```python
from build123d import *

# Parameters (mm, degrees)
F2_DEPTH  = 18.5
F3_R      = 1.55
F4_DEPTH  = 3.075
F5_W      = 6
F5_H      = 0.5
F6_DEPTH  = 0.2
F5_W_2    = 4
F5_H_2    = 2.25
F7_DEPTH  = 0.6
F8_W      = 4
F8_H      = 0.5
F9_DEPTH  = 0.9
F8_H_2    = 0.47
F10_DEPTH = 0.2
F11_W     = 4
F11_H     = 0.5
F12_DEPTH = 0.9
F11_H_2   = 0.47
F13_DEPTH = 0.2
F14_W     = 4
F14_H     = 0.5
F15_DEPTH = 0.7
F16_W     = 8
F16_H     = 7
F17_DEPTH = 1
F17_TAPER = 45
F18_W     = 8
F18_H     = 7
F19_DEPTH = 1
F19_TAPER = 45
F22_DEPTH = 0.2
F23_ANGLE = 90


with BuildPart() as f2:
    # F1 (on Front) → F2 (new body)
    with BuildSketch(Plane.XZ):
        with BuildLine():
            Line((-33.5725, -6), (33.5725, -6))
            ThreePointArc((33.5725, -6), (34.6331601718, -5.5606601718), (35.0725, -4.5))
            Line((35.0725, -4.5), (35.0725, 4.5))
            ThreePointArc((35.0725, 4.5), (34.6331601718, 5.5606601718), (33.5725, 6))
            Line((33.5725, 6), (-33.5725, 6))
            ThreePointArc((-33.5725, 6), (-34.6331601718, 5.5606601718), (-35.0725, 4.5))
            Line((-35.0725, 4.5), (-35.0725, -4.5))
            ThreePointArc((-35.0725, -4.5), (-34.6331601718, -5.5606601718), (-33.5725, -6))
        make_face()
        with BuildLine():
            ThreePointArc((-14.9225, -0.925), (-15.5082864376, -2.3392135624), (-16.9225, -2.925))
            Line((-16.9225, -2.925), (-30.0725, -2.925))
            ThreePointArc((-30.0725, -2.925), (-31.4867135624, -2.3392135624), (-32.0725, -0.925))
            Line((-32.0725, -0.925), (-32.0725, 0.925))
            ThreePointArc((-32.0725, 0.925), (-31.4867135624, 2.3392135624), (-30.0725, 2.925))
            Line((-30.0725, 2.925), (-16.9225, 2.925))
            ThreePointArc((-16.9225, 2.925), (-15.5082864376, 2.3392135624), (-14.9225, 0.925))
            Line((-14.9225, 0.925), (-14.9225, -0.925))
        make_face(mode=Mode.SUBTRACT)
        with BuildLine():
            Line((-9.6675, 4.265), (-1.0875, 4.265))
            ThreePointArc((-1.0875, 4.265), (-0.0268398282, 3.8256601718), (0.4125, 2.765))
            Line((0.4125, 2.765), (0.4125, -2.765))
            ThreePointArc((0.4125, -2.765), (-0.0268398282, -3.8256601718), (-1.0875, -4.265))
            Line((-1.0875, -4.265), (-9.6675, -4.265))
            ThreePointArc((-9.6675, -4.265), (-10.7281601718, -3.8256601718), (-11.1675, -2.765))
            Line((-11.1675, -2.765), (-11.1675, 2.765))
            ThreePointArc((-11.1675, 2.765), (-10.7281601718, 3.8256601718), (-9.6675, 4.265))
        make_face(mode=Mode.SUBTRACT)
        with BuildLine():
            Line((4.3325, 4.265), (12.9125, 4.265))
            ThreePointArc((12.9125, 4.265), (13.9731601718, 3.8256601718), (14.4125, 2.765))
            Line((14.4125, 2.765), (14.4125, -2.765))
            ThreePointArc((14.4125, -2.765), (13.9731601718, -3.8256601718), (12.9125, -4.265))
            Line((12.9125, -4.265), (4.3325, -4.265))
            ThreePointArc((4.3325, -4.265), (3.2718398282, -3.8256601718), (2.8325, -2.765))
            Line((2.8325, -2.765), (2.8325, 2.765))
            ThreePointArc((2.8325, 2.765), (3.2718398282, 3.8256601718), (4.3325, 4.265))
        make_face(mode=Mode.SUBTRACT)
        with BuildLine():
            ThreePointArc((32.0725, -3.8), (32.0139213562, -3.9414213562), (31.8725, -4))
            Line((31.8725, -4), (17.0725, -4))
            ThreePointArc((17.0725, -4), (16.9310786438, -3.9414213562), (16.8725, -3.8))
            Line((16.8725, -3.8), (16.8725, 3.8))
            ThreePointArc((16.8725, 3.8), (16.9310786438, 3.9414213562), (17.0725, 4))
            Line((17.0725, 4), (31.8725, 4))
            ThreePointArc((31.8725, 4), (32.0139213562, 3.9414213562), (32.0725, 3.8))
            Line((32.0725, 3.8), (32.0725, -3.8))
        make_face(mode=Mode.SUBTRACT)
    extrude(amount=-F2_DEPTH)

    # F3 (on face) → F4 (cut, through all)
    with BuildSketch(Plane.XY.offset(6)):
        with Locations((-23.4975, 13.2)):
            Circle(F3_R)
    extrude(amount=-F4_DEPTH, mode=Mode.SUBTRACT)

    # F5 (on face) → F6 (join)
    with BuildSketch(Plane.XY.offset(-2.925)):
        with Locations((-23.4975, 18.25)):
            Rectangle(F5_W, F5_H)
    extrude(amount=F6_DEPTH)

    # F5 (on face) → F7 (join)
    with BuildSketch(Plane.XY.offset(-2.925)):
        with Locations((-23.4975, 6.575)):
            Rectangle(F5_W_2, F5_H_2)
    extrude(amount=F7_DEPTH)

    # F8 (on face) → F9 (join)
    with BuildSketch(Plane.XY.offset(-4.265)):
        with Locations((-5.3775, 18.25)):
            Rectangle(F8_W, F8_H)
    extrude(amount=F9_DEPTH)

    # F8 (on face) → F10 (join)
    with BuildSketch(Plane.XY.offset(-4.265)):
        with Locations((-5.3775, 0.235)):
            Rectangle(F8_W, F8_H_2)
    extrude(amount=F10_DEPTH)

    # F11 (on face) → F12 (join)
    with BuildSketch(Plane.XY.offset(-4.265)):
        with Locations((8.6225, 18.25)):
            Rectangle(F11_W, F11_H)
    extrude(amount=F12_DEPTH)

    # F11 (on face) → F13 (join)
    with BuildSketch(Plane.XY.offset(-4.265)):
        with Locations((8.6225, 0.235)):
            Rectangle(F11_W, F11_H_2)
    extrude(amount=F13_DEPTH)

    # F14 (on face) → F15 (join)
    with BuildSketch(Plane.XY.offset(-4)):
        with Locations((24.4725, 18.25)):
            Rectangle(F14_W, F14_H)
    extrude(amount=F15_DEPTH)

    # F16 (on face) → F17 (cut)
    with BuildSketch(Plane.YZ.offset(35.0725)):
        with Locations((9.25, 0)):
            Rectangle(F16_W, F16_H)
    extrude(amount=-F17_DEPTH, taper=F17_TAPER, mode=Mode.SUBTRACT)

    # F18 (on face) → F19 (cut)
    with BuildSketch(Plane(origin=(-35.0725, 0, 0), x_dir=(0, -1, 0), z_dir=(-1, 0, 0))):
        with Locations((-9.25, 0)):
            Rectangle(F18_W, F18_H)
    extrude(amount=-F19_DEPTH, taper=F19_TAPER, mode=Mode.SUBTRACT)

    # F21 (on face) → F22 (join)
    with BuildSketch(Plane(origin=(0, 18.5, 0), x_dir=(-1, 0, 0), z_dir=(0, 1, 0))):
        with BuildLine():
            Line((-33.5725, 6), (-31.6655044446, 6))
            ThreePointArc((-31.6655044446, 6), (-36.7544805153, 7.6819805153), (-35.0725, 2.5930044446))
            Line((-35.0725, 2.5930044446), (-35.0725, 4.5))
            ThreePointArc((-35.0725, 4.5), (-34.6331601718, 5.5606601718), (-33.5725, 6))
        make_face()
        with BuildLine():
            Line((-35.0725, -4.5), (-35.0725, -2.5930044446))
            ThreePointArc((-35.0725, -2.5930044446), (-36.7544805153, -7.6819805153), (-31.6655044446, -6))
            Line((-31.6655044446, -6), (-33.5725, -6))
            ThreePointArc((-33.5725, -6), (-34.6331601718, -5.5606601718), (-35.0725, -4.5))
        make_face()
        with BuildLine():
            ThreePointArc((37.6331601718, 5.5606601718), (34.8534245792, 8.5525631767), (31.6655044446, 6))
            Line((31.6655044446, 6), (33.5725, 6))
            ThreePointArc((33.5725, 6), (34.6331601718, 5.5606601718), (35.0725, 4.5))
            Line((35.0725, 4.5), (35.0725, 2.5930044446))
            ThreePointArc((35.0725, 2.5930044446), (36.9045055313, 3.6008157245), (37.6331601718, 5.5606601718))
        make_face()
        with BuildLine():
            ThreePointArc((37.6331601718, -5.5606601718), (36.9045055313, -3.6008157245), (35.0725, -2.5930044446))
            Line((35.0725, -2.5930044446), (35.0725, -4.5))
            ThreePointArc((35.0725, -4.5), (34.6331601718, -5.5606601718), (33.5725, -6))
            Line((33.5725, -6), (31.6655044446, -6))
            ThreePointArc((31.6655044446, -6), (34.8534245792, -8.5525631767), (37.6331601718, -5.5606601718))
        make_face()
    extrude(amount=-F22_DEPTH)


with BuildPart() as f2_1:
    # F23: moved
    add(f2.part.rotate(Axis((0, 18.5, 6), (-1, 0, 0)), F23_ANGLE))


solid = f2_1.part
```
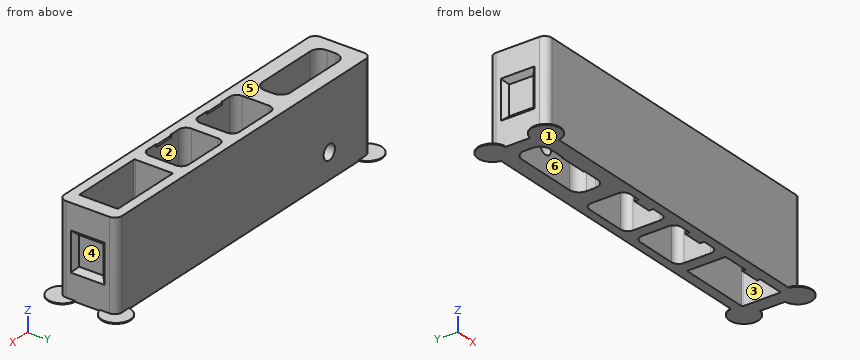
Could you check a few things on this model? Use its own coordinates, in mm. Face numbers are marked on the shaded views. A direction names the side the tool comes from. Round coordinates to 2 decimals unless told otherwise and drop trailing zeros. Loops run counter-clockwise (first coordinate to the right, second up) from the corner with the lowest first, then second, coordinate; pieces in that order, holes last. Notation, with made-up numbers: (86, 33.5) - (100, 33.5) arc R20 cw to (100, 72.5) - close; hole circle Ø3 at (42.25, 33.5). An arc over 180 degrees is marked (long way). Answer in a Markdown table with one row per item. Add a question column.
(1) For the marked faces 1, 2 and 3, which set-ups out of +Z, -Z, +X, -X, +Y, -Y let a thin tool reach every point of the face, with its end or its side?
(2) I'm going to push flat-ended pins straight in: pin 1 (9.5 mm diameter, centred on x = 6.5, z = 11, fed in from +Y); pin 2 (7.5 mm diameter, centred on x = 27, z = 19.5, fed in from -Y); pin 3 (6 mm diameter, centred on y = 6, z = 19.5, fed in from -X). Where does each tip first touch, or does it pass through?
(3) If we section it at B-B (x = 5): Please give me the cut outline in (y, z) (3 decimals).
(4) If we section it at C-C (z = 22.75): State how many separate pieces and enclosed holes the cut face has, plus the area to 3 significant figures.
(5) I need wall thicknesses on line 1 along X through (y, z) = (13.25, 17.25); line 2 along X through (y, z) = (10.25, 14.5); line 3 along Y through (x, z) = (-1.5, 21.25) (3 decimals). Which ranges of each line are inside material? Lowest first, please.
(6) If we section it at A-A (x = 30.5): Please give me the cut outline in (y, z), plus the area to 3 significant figures.
(7) If we mould it in two halves opening along X, with no side actions, what happens to the marked faces 4, 5 and 6? For each: pulls with the +X half, pulls with the -X half, needs draft (parallel to the pull), parting line crosses it, or undercut.
Model answer:
| question | item | result |
|---|---|---|
| 1 | face 1 | -Z, +X, -X, +Y, -Y |
| 1 | face 2 | none |
| 1 | face 3 | +Z, -Z |
| 2 | pin 1 | stops at y = 18.5 |
| 2 | pin 2 | stops at y = 6.5 |
| 2 | pin 3 | stops at x = -35.07 |
| 3 | outline | (6.5, 6) - (8.235, 6) - (8.235, 24.5) - (6.5, 24.5) - close; (16.765, 6) - (18.5, 6) - (18.5, 24.5) - (16.765, 24.5) - close |
| 4 | separate pieces | 1 |
| 4 | enclosed holes | 4 |
| 4 | area | 428 mm² |
| 5 | line 1 | x = -34.07 to -32.07, -14.92 to -11.17, 0.41 to 2.83, 14.41 to 16.87, 32.07 to 34.07 |
| 5 | line 2 | x = -34.07 to -31.57, -15.42 to -11.17, 0.41 to 2.83, 14.41 to 16.87, 32.07 to 34.07 |
| 5 | line 3 | y = 6.5 to 8.235, 16.765 to 18.5 |
| 6 | outline | (6.5, 6) - (8.5, 6) - (8.5, 24.5) - (6.5, 24.5) - close; (16.5, 6) - (18.5, 6) - (18.5, 24.5) - (16.5, 24.5) - close |
| 6 | area | 74.0 mm² |
| 7 | face 4 | pulls with the +X half |
| 7 | face 5 | needs draft |
| 7 | face 6 | undercut |
